Print and shaded views of the part. All mm, measured from the part's lowest x, y and z. Round coordinates to 2 decimals unless told otherwise and drop trailing zeros. Write each loop counter-clockwise with the first axis right and the second up, starting at its lowest first coordinate (ties: lowest second). Pieces come first, ordered by that corner, then holes.
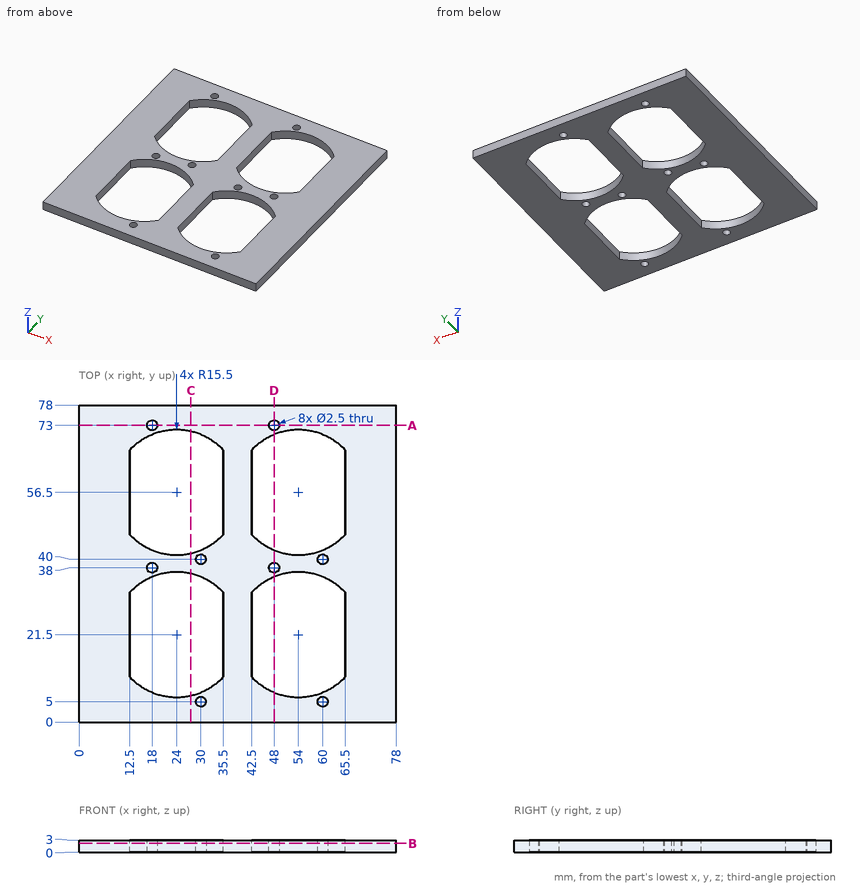
1) Slice it at C-C (x = 27.5). Write the cut outline in (y, z).
Results:
outline: (0, 0) - (6.4, 0) - (6.4, 3) - (0, 3) - close; (36.6, 0) - (41.4, 0) - (41.4, 3) - (36.6, 3) - close; (71.6, 0) - (78, 0) - (78, 3) - (71.6, 3) - close
2) Wall check: L1, parallel to X at y = 73, z = 1.8; L2, parallel to X at y = 48, z = 0.15; L3, parallel to Y at x = 60, z = 1.3. Give the ranges that are in metal, low to high.
Results:
L1: x = 0 to 16.75, 19.25 to 46.75, 49.25 to 78
L2: x = 0 to 12.5, 35.5 to 42.5, 65.5 to 78
L3: y = 0 to 3.75, 6.25 to 7.21, 35.79 to 38.75, 41.25 to 42.21, 70.79 to 78
3) Slice it at A-A (y = 73). Write the cut outline in (x, z), plus the area to 3 significant figures.
Results:
outline: (0, 0) - (16.75, 0) - (16.75, 3) - (0, 3) - close; (19.25, 0) - (46.75, 0) - (46.75, 3) - (19.25, 3) - close; (49.25, 0) - (78, 0) - (78, 3) - (49.25, 3) - close
area: 219 mm2
4) Slice it at B-B (z = 2.15). Count the separate pieces of the cut face and the enclosed holes in it, plus the area to 3 significant figures.
Results:
separate pieces: 1
enclosed holes: 12
area: 3,480 mm2
5) Slice it at D-D (x = 48). Write the cut outline in (y, z), plus the area to 3 significant figures.
Results:
outline: (0, 0) - (7.21, 0) - (7.21, 3) - (0, 3) - close; (35.79, 0) - (36.75, 0) - (36.75, 3) - (35.79, 3) - close; (39.25, 0) - (42.21, 0) - (42.21, 3) - (39.25, 3) - close; (70.79, 0) - (71.75, 0) - (71.75, 3) - (70.79, 3) - close; (74.25, 0) - (78, 0) - (78, 3) - (74.25, 3) - close
area: 47.5 mm2
